Model file for the job. Use its own axes, mm. A direction names the side the tool comes from. Give positions to 0.01 mm unless a question says otherwise; leave off trailing zeros. Loops run counter-clockwise (first coordinate to the right, second up) from the corner with the lowest first, then second, coordinate; pieces in that order, holes last. Notation, with made-up numbers: (-14.5, 19) - (9.5, 19) arc R7 ccw to (9.5, 31) - close; hole circle Ø7 at (-26.5, -6). An arc over 180 degrees is marked (long way). Use a Markdown table: item, result.
from build123d import *

# Parameters (mm, degrees)
SKETCH_1_W           = 70
SKETCH_1_H           = 5
EXTRUDE_1_DEPTH      = 8
SKETCH_3_W           = 38
SKETCH_3_H           = 5
EXTRUDE_2_DEPTH      = 43
SKETCH_4_W           = 38
SKETCH_4_H           = 5
EXTRUDE_3_DEPTH      = 45
SKETCH_5_R           = 11.5
SKETCH_5_R_2         = 1.6
CUT_EXTRUDE_2_DEPTH  = 45
FILLET_1_R           = 5
CUT_EXTRUDE_3_REACH  = 81.536
SKETCH_6_W           = 42
SKETCH_6_H           = 1.562526182
EXTRUDE_4_DEPTH      = 7
EXTRUDE_4_DEPTH_BACK = 45
SKETCH_7_W           = 13.004753842
SKETCH_7_H           = 5
FILLET_2_R           = 10
SKETCH_13_W          = 70
SKETCH_13_H          = 47.548344346
EXTRUDE_6_DEPTH      = 5
SKETCH_10_R          = 2.5
CUT_EXTRUDE_6_DEPTH  = 10
SKETCH_11_W          = 40
SKETCH_11_H          = 5
EXTRUDE_5_DEPTH      = 29
SKETCH_12_R          = 1.6
CUT_EXTRUDE_7_DEPTH  = 7
SKETCH_14_R          = 1.6
CUT_EXTRUDE_8_DEPTH  = 7
SKETCH_15_R          = 3.15
CUT_EXTRUDE_9_DEPTH  = 3.5
FILLET_3_R           = 10
SKETCH_16_R          = 1.6
CUT_EXTRUDE_10_DEPTH = 10


with BuildPart() as part:
    # 草图1 → 凸台-拉伸1 (new body)
    with BuildSketch(Plane.XY):
        Rectangle(SKETCH_1_W, SKETCH_1_H)
    extrude(amount=EXTRUDE_1_DEPTH)

    # 草图3 → 凸台-拉伸2 (add)
    with BuildSketch(Plane.XY.offset(8)):
        Rectangle(SKETCH_3_W, SKETCH_3_H)
    extrude(amount=EXTRUDE_2_DEPTH)

    # 草图4 → 凸台-拉伸3 (add)
    with BuildSketch(Plane(origin=(0, 2.5, 0), x_dir=(1, 0, 0), z_dir=(0, 1, 0))):
        with Locations((0, -48.5)):
            Rectangle(SKETCH_4_W, SKETCH_4_H)
    extrude(amount=EXTRUDE_3_DEPTH)

    # 草图5 → 切除-拉伸2 (cut)
    with BuildSketch(Plane.XY.offset(51)):
        with Locations((0, 23.5)):
            Circle(SKETCH_5_R)
        with Locations((-15.25, 38.75)):
            Circle(SKETCH_5_R_2)
        with Locations((15.25, 38.75)):
            Circle(SKETCH_5_R_2)
        with Locations((-15.25, 8.25)):
            Circle(SKETCH_5_R_2)
        with Locations((15.25, 8.25)):
            Circle(SKETCH_5_R_2)
    extrude(amount=-CUT_EXTRUDE_2_DEPTH, mode=Mode.SUBTRACT)

    # 圆角1
    fillet_1_edges = [part.edges().sort_by_distance(p)[0] for p in [
        (-19, 47.5, 48.5),
        (19, 47.5, 48.5),
    ]]
    fillet(fillet_1_edges, radius=FILLET_1_R)

    # 切除-拉伸3: up to this face of the body (flat: up to its plane)
    cut_extrude_3_end = Plane(part.part.faces().sort_by_distance((0, 2.5, 20.572854291))[0])
    # 草图6 → 切除-拉伸3 (cut, up to the picked face)
    with BuildSketch(Plane(origin=(0, 47.5, 0), x_dir=(1, 0, 0), z_dir=(0, 1, 0)), mode=Mode.PRIVATE) as cut_extrude_3_sk1:
        with Locations((0, -46.703490751)):
            Rectangle(SKETCH_6_W, SKETCH_6_H)
    cut_extrude_3_tool1 = split(extrude(cut_extrude_3_sk1.sketch, amount=-CUT_EXTRUDE_3_REACH, mode=Mode.PRIVATE), bisect_by=cut_extrude_3_end, keep=Keep.BOTH, mode=Mode.PRIVATE)
    add(cut_extrude_3_tool1.solids().sort_by(Axis((0, 47.5, 46.703491), (0, -1, 0)))[0], mode=Mode.SUBTRACT)

    # 草图7 → 凸台-拉伸4 (add, two sides: drawn at the far end of the back side and taken through both)
    with BuildSketch(Plane(origin=(19, 0, 0), x_dir=(0, 0, -1), z_dir=(1, 0, 0)).offset(-EXTRUDE_4_DEPTH_BACK)):
        with Locations((-44.497623079, 0)):
            Rectangle(SKETCH_7_W, SKETCH_7_H)
    extrude(amount=EXTRUDE_4_DEPTH + EXTRUDE_4_DEPTH_BACK)

    # 圆角2
    # the kernel refuses this fillet: 10 mm, written as the material it adds along each edge
    with BuildSketch(Plane(origin=(-19, 2.5, 47.484753842), x_dir=(-1, 0, 0), z_dir=(0, 0, 1)), Plane(origin=(19, 2.5, 51), x_dir=(1, 0, 0), z_dir=(0, 0, -1))) as fillet_2_piece_1:
        with BuildLine():
            CenterArc((10, -9.539392014), FILLET_2_R, 107.457603124, 72.542396876)
            Line((0, -9.539392014), (-0.2, -9.539392014))
            Line((-0.2, -9.539392014), (-0.2, 0))
            Line((-0.2, 0), (0, 0.2))
            ThreePointArc((0, 0.2), (3.5, 0.2), (6.94, 0.19078784))
            Line((6.94, 0.19078784), (7, 0))
        make_face()
    extrude(amount=3.515246158)

    # 草图13 → 凸台-拉伸6 (add)
    with BuildSketch(Plane(origin=(0, 2.5, 0), x_dir=(1, 0, 0), z_dir=(0, 1, 0))):
        with Locations((0, -23.742376921)):
            Rectangle(SKETCH_13_W, SKETCH_13_H)
    extrude(amount=-EXTRUDE_6_DEPTH)

    # 草图10 → 切除-拉伸6 (cut)
    with BuildSketch(Plane.XY.offset(51)):
        with Locations((-15.25, 38.75)):
            Circle(SKETCH_10_R)
        with Locations((15.25, 38.75)):
            Circle(SKETCH_10_R)
        with Locations((15.25, 8.25)):
            Circle(SKETCH_10_R)
        with Locations((-15.25, 8.25)):
            Circle(SKETCH_10_R)
    extrude(amount=-CUT_EXTRUDE_6_DEPTH, mode=Mode.SUBTRACT)

    # 草图11 → 凸台-拉伸5 (add)
    with BuildSketch(Plane.XY.offset(51)):
        Rectangle(SKETCH_11_W, SKETCH_11_H)
    extrude(amount=EXTRUDE_5_DEPTH)

    # 草图12 → 切除-拉伸7 (cut)
    with BuildSketch(Plane(origin=(0, 2.5, 0), x_dir=(1, 0, 0), z_dir=(0, 1, 0))):
        with Locations(Location((15, -76, 0), (0, 0, 180))):
            Circle(SKETCH_12_R)
        with Locations(Location((-15, -76, 0), (0, 0, 180))):
            Circle(SKETCH_12_R)
    extrude(amount=-CUT_EXTRUDE_7_DEPTH, mode=Mode.SUBTRACT)

    # 草图14 → 切除-拉伸8 (cut)
    with BuildSketch(Plane(origin=(0, 2.5, 0), x_dir=(1, 0, 0), z_dir=(0, 1, 0))):
        with Locations(Location((28, -7, 0), (0, 0, 270))):
            Circle(SKETCH_14_R)
        with Locations(Location((-28, -7, 0), (0, 0, 270))):
            Circle(SKETCH_14_R)
    extrude(amount=-CUT_EXTRUDE_8_DEPTH, mode=Mode.SUBTRACT)

    # 草图15 → 切除-拉伸9 (cut)
    with BuildSketch(Plane(origin=(0, 2.5, 0), x_dir=(1, 0, 0), z_dir=(0, 1, 0))):
        with Locations(Location((28, -7, 0), (0, 0, 270))):
            Circle(SKETCH_15_R)
        with Locations(Location((-28, -7, 0), (0, 0, 270))):
            Circle(SKETCH_15_R)
    extrude(amount=-CUT_EXTRUDE_9_DEPTH, mode=Mode.SUBTRACT)

    # 圆角3
    fillet_3_edges = [part.edges().sort_by_distance(p)[0] for p in [
        (35, 0, -0.031795252),
        (-35, 0, -0.031795252),
    ]]
    fillet(fillet_3_edges, radius=FILLET_3_R)

    # 草图16 → 切除-拉伸10 (cut)
    with BuildSketch(Plane(origin=(0, 2.5, 0), x_dir=(1, 0, 0), z_dir=(0, 1, 0))):
        with Locations(Location((31.5, -32.518590997, 0), (0, 0, 270))):
            Circle(SKETCH_16_R)
        with Locations(Location((31.5, -12.518590997, 0), (0, 0, 270))):
            Circle(SKETCH_16_R)
        with Locations(Location((-31.5, -32.518590997, 0), (0, 0, 270))):
            Circle(SKETCH_16_R)
        with Locations(Location((-31.5, -12.518590997, 0), (0, 0, 270))):
            Circle(SKETCH_16_R)
    extrude(amount=-CUT_EXTRUDE_10_DEPTH, mode=Mode.SUBTRACT)


solid = part.part
(1) Slice it at B-B, the plane x = 10. Write the cut outline in (y, z).
Computed:
| item | result |
|---|---|
| outline | (-2.5, -0.03) - (2.5, -0.03) - (2.5, 47.48) - (17.82, 47.48) - (17.82, 51) - (2.5, 51) - (2.5, 80) - (-2.5, 80) - close; (29.18, 47.48) - (47.5, 47.48) - (47.5, 51) - (29.18, 51) - close |
(2) Slice it at D-D, the plane x = -6. Write the cut outline in (y, z).
Computed:
| item | result |
|---|---|
| outline | (-2.5, -0.03) - (2.5, -0.03) - (2.5, 47.48) - (13.69, 47.48) - (13.69, 51) - (2.5, 51) - (2.5, 80) - (-2.5, 80) - close; (33.31, 47.48) - (47.5, 47.48) - (47.5, 51) - (33.31, 51) - close |
(3) Pin check, flat tips, straight feed: P1, Ø4, axis at x = 31.5, z = 32.52, coming from the +Y side; P2, Ø1.7, axis at y = 0.5, z = 48.5, coming from the +X side; P3, Ø3, axis at y = 1, z = 50, coming from the -X side. Stop position of each tip, or through.
Computed:
| item | result |
|---|---|
| P1 | y = 2.5 |
| P2 | x = 26 |
| P3 | x = -26 |
(4) 3-axis set-ups, long thin cutter, end or side, ignore diameter. For faces 4 (the flat face through (0, 47.5, 49)), 5 (the flat face through (-19, 27, 49)), 6 (the cylindrical face through (26.79, 0.77, 9.91)), 7 (the cylindrical face through (30.9, 0, 14)), 8 (the flat face through (20, 0, 65)): which of +Z, -Z, +X, -X, +Y, -Y reach the whole face in a straight line?
Computed:
| item | result |
|---|---|
| face 4 | +Z, -Z, +X, -X, +Y |
| face 5 | +Z, -Z, -X, +Y |
| face 6 | +Y |
| face 7 | +Y, -Y |
| face 8 | +Z, +X, +Y, -Y |
(5) Mould opens along Y. For faces 1 (the flat face through (19, 27, 49)), 2 (the cylindrical face through (17.5, 46.07, 49.22)), 3 (the cylindrical face through (-1.5, 34.9, 49.3)) say: pulls with the +Y half, pulls with the -Y half, needs draft (parallel to the pull), parting line crosses it, or undercut.
Computed:
| item | result |
|---|---|
| face 1 | needs draft |
| face 2 | pulls with the +Y half |
| face 3 | undercut |
(6) Slice it at A-A, the plane y = 23.5. Write the cut outline in (x, z).
Computed:
| item | result |
|---|---|
| outline | (-19, 47.48) - (-11.5, 47.48) - (-11.5, 51) - (-19, 51) - close; (11.5, 47.48) - (19, 47.48) - (19, 51) - (11.5, 51) - close |
(7) Drill centre lines: probe 1 along Y at (x, z) = (0, 49); probe 2 along Y at (x, z) = (-24, 18); probe 3 along X at (y, z) = (13, 49). Where is each one in solid material? Low to high. Write a range as [from, to].
Computed:
| item | result |
|---|---|
| probe 1 | [-2.5, 12], [35, 47.5] |
| probe 2 | [-2.5, 2.5] |
| probe 3 | [-19, -4.69], [4.69, 19] |
(8) Slice it at C-C, the plane z = 7. Write the cut outline in (x, y), plus the area to 3 significant figures.
Computed:
| item | result |
|---|---|
| outline | (-34.55, -2.5) - (-29.6, -2.5) - (-29.6, -1) - (-31.15, -1) - (-31.15, 2.5) - (-34.55, 2.5) - close; (-26.4, -2.5) - (26.4, -2.5) - (26.4, -1) - (24.85, -1) - (24.85, 2.5) - (-24.85, 2.5) - (-24.85, -1) - (-26.4, -1) - close; (29.6, -2.5) - (34.55, -2.5) - (34.55, 2.5) - (31.15, 2.5) - (31.15, -1) - (29.6, -1) - close |
| area | 292 mm² |
